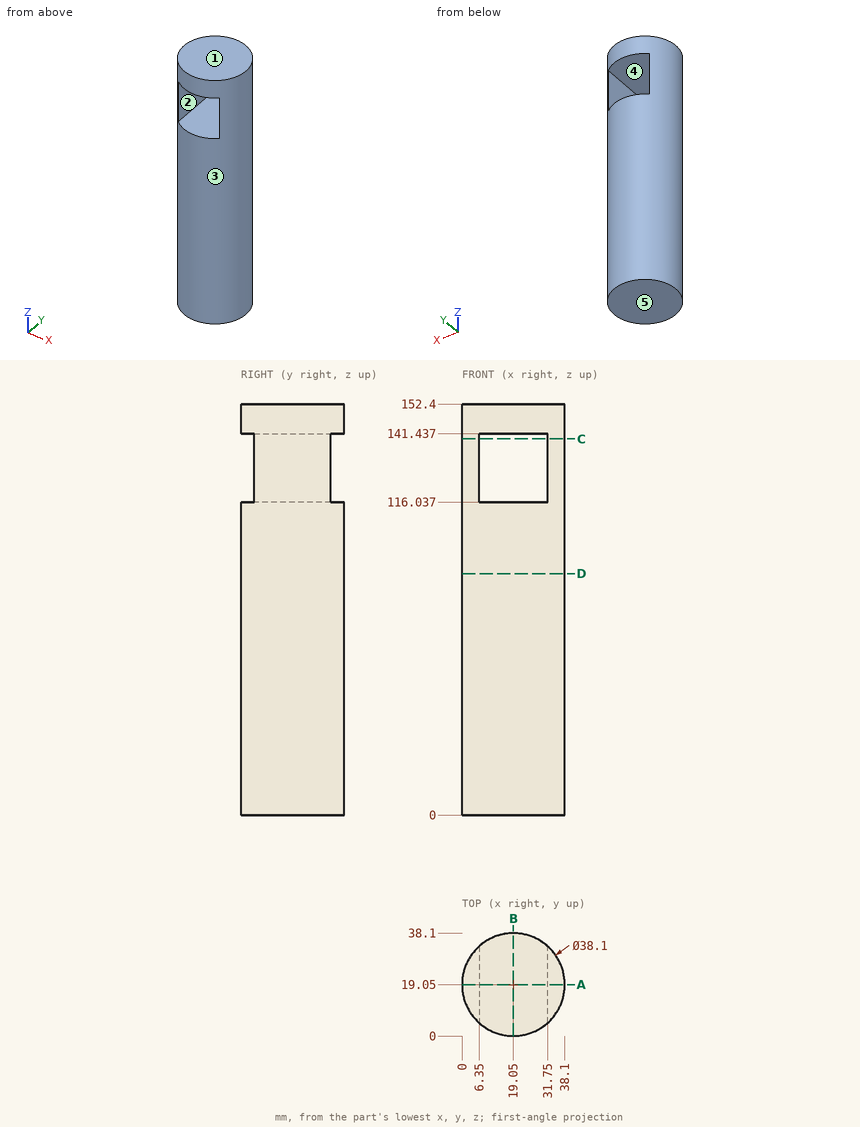
Verification items for this drawing (mm, ordinates from the low corner). A direction names the side the tool comes from. Coordinates: 2 decimals unless noted, no trailing zeros. Write each loop counter-clockwise with the first axis right and the second up, starting at its lowest first coordinate (ties: lowest second). Pieces come first, ordered by that corner, then holes. Notation, with made-up numbers: (38, -6) - (85, -6) arc R18 ccw to (85, -2) - close; hole circle Ø9 at (14, 1). An arc over 180 degrees is marked (long way). One line per question, with ' | ' between items.
Item 1: Gauge pin test, flat ends, axial feed: P1, Ø5, axis at y = 5.5, z = 104.5, coming from the -X side; P2, Ø10, axis at y = 30.5, z = 43, coming from the -X side (1 decimal); P3, Ø3, axis at y = 4, z = 65, coming from the -X side. Record the tip position at first contact, or that the pin passes through.
Determined:
P1: stops at x = 3.53 | P2: stops at x = 1.1 | P3: stops at x = 5.66
Item 2: Sectioned sample at A-A on y = 19.05. Record the boundary of the cut face in (x, z), plus the area to 3 significant figures.
Determined:
outline: (0, 0) - (38.1, 0) - (38.1, 152.4) - (0, 152.4) - close; hole (6.35, 116.04) - (31.75, 116.04) - (31.75, 141.44) - (6.35, 141.44) - close | area: 5,160 mm2
Item 3: Sectioned sample at D-D on z = 89.5. Record the boundary of the cut face in (x, y).
Determined:
outline: circle Ø38.1 at (19.05, 19.05)
Item 4: Thickness scan on line 1 (Z direction, x = 23.5, y = 36); line 2 (X direction, y = 18, z = 72); line 3 (X direction, y = 6, z = 117). Record the ranges inside material, lowest first. Write a range as [from, to].
Determined:
line 1: z = [0, 116.04], [141.44, 152.4] | line 2: x = [0.03, 38.07] | line 3: x = [5.17, 6.35], [31.75, 32.93]
Item 5: Mould release check, pull along X, two halves, no side actions. Record for the marked faces 3, 4 and 5: pulls with the +X half, pulls with the -X half, needs draft (parallel to the pull), parting line crosses it, or undercut.
Determined:
face 3: parting line crosses it | face 4: undercut | face 5: needs draft
Item 6: Sectioned sample at C-C on z = 139.5. Record the boundary of the cut face in (x, y), plus the area to 3 significant figures.
Determined:
outline: (6.35, 4.85) - (6.35, 33.25) arc R19.05 ccw to start; (31.75, 4.85) arc R19.05 ccw to (31.75, 33.25) - close | area: 250 mm2
Item 7: Access from +Z, -Z, +X, -X, +Y, -Y to the whole of each face (thin tool, end or side, straight path). Record for the marked faces 1 and 2.
Determined:
face 1: +Z, +X, -X, +Y, -Y | face 2: +Y, -Y
Item 8: Sectioned sample at B-B on x = 19.05. Record the boundary of the cut face in (y, z), plus the area to 3 significant figures.
Determined:
outline: (0, 0) - (38.1, 0) - (38.1, 116.04) - (0, 116.04) - close; (0, 141.44) - (38.1, 141.44) - (38.1, 152.4) - (0, 152.4) - close | area: 4,840 mm2
